Input: part model. Units: mm. Frame: model coordinates. A direction names the side the tool comes from. Round coordinates to 2 decimals unless told otherwise and drop trailing zeros. Order: outer loops, then holes, each group sorted by start corner. A loop starts at its lowest first (then second) coordinate and runs counter-clockwise, first axis right, second up. Notation, with made-up numbers: (57, 38) -> (91, 38) arc R25 cw to (91, 52) -> close; hole circle Ø2 at (11.25, 78). An arc over 180 degrees is marked (long way). Use a Markdown table: item, result.
from build123d import *

# Parameters (mm, degrees)
SKETCH_W                = 90
SKETCH_H                = 35
PAD_DEPTH               = 3
SKETCH001_R             = 10.5
HOLE_DEPTH              = 25
HOLE_TEARDROPS_DEPTH    = 25
SKETCH002_R             = 4
PAD001_DEPTH            = 5.6
POCKET_DEPTH            = 5.6
SKETCH004_R             = 1.45
HOLE001_DEPTH           = 25
HOLE001_TEARDROPS_DEPTH = 25
FILLET_R                = 2
CHAMFER_SIZE            = 0.4
FILLET001_R             = 1
PAD002_DEPTH            = 7
SKETCH005_R             = 14.71653
PAD003_DEPTH            = 10
SKETCH006_R             = 4.05
PAD004_DEPTH            = 5.6
POCKET001_DEPTH         = 5.6
SKETCH008_R             = 1.45
HOLE002_DEPTH           = 25
HOLE002_TEARDROPS_DEPTH = 25
FILLET002_R             = 2
CHAMFER001_SIZE         = 0.4
POCKET002_DEPTH         = 7
CHAMFER002_SIZE         = 0.4
CHAMFER003_SIZE         = 0.6


with BuildPart() as part:
    # Sketch → Pad (new body)
    with BuildSketch(Plane.XY):
        Rectangle(SKETCH_W, SKETCH_H)
    extrude(amount=PAD_DEPTH)

    # Sketch001 (on Face6 of Pad) → Hole (cut)
    with BuildSketch(Plane.XY.offset(3)):
        with Locations((-12, 0)):
            Circle(SKETCH001_R)
    extrude(amount=-HOLE_DEPTH, mode=Mode.SUBTRACT)

    # Sketch001_Teardrops (on Sketch) → Hole_Teardrops (cut)
    with BuildSketch(Plane.XY.offset(3)):
        with BuildLine():
            ThreePointArc((-17.25, 9.093267), (-12, -10.5), (-6.75, 9.093267))
            Line((-6.75, 9.093267), (-12, 12.124356))
            Line((-17.25, 9.093267), (-12, 12.124356))
        make_face()
    extrude(amount=-HOLE_TEARDROPS_DEPTH, mode=Mode.SUBTRACT)

    # Sketch002 (on Face5 of Hole_Teardrops) → Pad001 (join)
    with BuildSketch(Plane.XY.offset(3)):
        with Locations((35, 0)):
            Circle(SKETCH002_R)
        with Locations((12, 0)):
            Circle(SKETCH002_R)
        with Locations((-35, 0)):
            Circle(SKETCH002_R)
    extrude(amount=PAD001_DEPTH)

    # Sketch003 (on Face13 of Pad001) → Pocket (cut)
    with BuildSketch(Plane.XY.offset(8.6)):
        Polygon((-35, 3), (-38.464102, 5), (-31.535898, 5), align=None)
        Polygon((12, 3), (8.535898, 5), (15.464102, 5), align=None)
        Polygon((38.464102, 5), (35, 3), (31.535898, 5), align=None)
    extrude(amount=-POCKET_DEPTH, mode=Mode.SUBTRACT)

    # Sketch004 (on Face17 of Pocket) → Hole001 (cut)
    with BuildSketch(Plane.XY.offset(8.6)):
        with Locations((-35, 0)):
            Circle(SKETCH004_R)
        with Locations((12, 0)):
            Circle(SKETCH004_R)
        with Locations((35, 0)):
            Circle(SKETCH004_R)
    extrude(amount=-HOLE001_DEPTH, mode=Mode.SUBTRACT)

    # Sketch004_Teardrops (on Sketch) → Hole001_Teardrops (cut)
    with BuildSketch(Plane.XY.offset(8.6)):
        with BuildLine():
            ThreePointArc((-35.725, 1.255737), (-35, -1.45), (-34.275, 1.255737))
            Line((-34.275, 1.255737), (-35, 1.674316))
            Line((-35.725, 1.255737), (-35, 1.674316))
        make_face()
        with BuildLine():
            ThreePointArc((11.275, 1.255737), (12, -1.45), (12.725, 1.255737))
            Line((12.725, 1.255737), (12, 1.674316))
            Line((11.275, 1.255737), (12, 1.674316))
        make_face()
        with BuildLine():
            ThreePointArc((34.275, 1.255737), (35, -1.45), (35.725, 1.255737))
            Line((35.725, 1.255737), (35, 1.674316))
            Line((34.275, 1.255737), (35, 1.674316))
        make_face()
    extrude(amount=-HOLE001_TEARDROPS_DEPTH, mode=Mode.SUBTRACT)

    # Fillet
    fillet_edges = [part.edges().sort_by_distance(p)[0] for p in [
        (36.334875, 3.770691, 5.8),
        (33.665125, 3.770691, 5.8),
        (13.334875, 3.770691, 5.8),
        (10.665125, 3.770691, 5.8),
        (-33.665125, 3.770691, 5.8),
        (-36.334875, 3.770691, 5.8),
    ]]
    fillet(fillet_edges, radius=FILLET_R)

    # Chamfer
    chamfer_edges = [part.edges().sort_by_distance(p)[0] for p in [
        (33.392214, -3.662653, 8.6),
        (10.392214, -3.662653, 8.6),
        (-36.607786, -3.662653, 8.6),
        (-35.725, -1.255737, 8.6),
        (11.275, -1.255737, 8.6),
        (34.275, -1.255737, 8.6),
    ]]
    chamfer(chamfer_edges, length=CHAMFER_SIZE)

    # Fillet001
    fillet001_edges = [part.edges().sort_by_distance(p)[0] for p in [
        (45, 17.5, 1.5),
        (-45, 17.5, 1.5),
        (-45, -17.5, 1.5),
        (45, -17.5, 1.5),
    ]]
    fillet(fillet001_edges, radius=FILLET001_R)

    # Fillet001 Face28 → Pad002 (add)
    with BuildSketch(Plane(origin=(1.493435, -0.023344, 0), x_dir=(0, -1, 0), z_dir=(0, 0, -1))):
        with BuildLine():
            Line((16.476656, 46.493435), (-16.523344, 46.493435))
            ThreePointArc((-16.523344, 46.493435), (-17.230451, 46.200542), (-17.523344, 45.493435))
            Line((-17.523344, 45.493435), (-17.523344, -42.506565))
            ThreePointArc((-17.523344, -42.506565), (-17.230451, -43.213672), (-16.523344, -43.506565))
            Line((-16.523344, -43.506565), (16.476656, -43.506565))
            ThreePointArc((16.476656, -43.506565), (17.183762, -43.213672), (17.476656, -42.506565))
            Line((17.476656, -42.506565), (17.476656, 45.493435))
            ThreePointArc((17.476656, 45.493435), (17.183762, 46.200542), (16.476656, 46.493435))
        make_face()
        with BuildLine():
            ThreePointArc((-0.023344, 35.043435), (-0.748344, 35.237698), (-1.279081, 35.768435))
            Line((-1.279081, 35.768435), (-1.69766, 36.493435))
            Line((-1.69766, 36.493435), (-1.279081, 37.218435))
            ThreePointArc((-1.279081, 37.218435), (1.232392, 37.218435), (-0.023344, 35.043435))
        make_face(mode=Mode.SUBTRACT)
        with BuildLine():
            ThreePointArc((-0.023344, -11.956565), (-0.748344, -11.762302), (-1.279081, -11.231565))
            Line((-1.279081, -11.231565), (-1.69766, -10.506565))
            Line((-1.69766, -10.506565), (-1.279081, -9.781565))
            ThreePointArc((-1.279081, -9.781565), (1.232392, -9.781565), (-0.023344, -11.956565))
        make_face(mode=Mode.SUBTRACT)
        with BuildLine():
            ThreePointArc((-0.023344, -34.956565), (-0.748344, -34.762302), (-1.279081, -34.231565))
            Line((-1.279081, -34.231565), (-1.69766, -33.506565))
            Line((-1.69766, -33.506565), (-1.279081, -32.781565))
            ThreePointArc((-1.279081, -32.781565), (1.232392, -32.781565), (-0.023344, -34.956565))
        make_face(mode=Mode.SUBTRACT)
        with BuildLine():
            ThreePointArc((-0.023344, 2.993435), (-5.273344, 4.400168), (-9.116611, 8.243435))
            Line((-9.116611, 8.243435), (-12.1477, 13.493435))
            Line((-12.1477, 13.493435), (-9.116611, 18.743435))
            ThreePointArc((-9.116611, 18.743435), (9.069922, 18.743435), (-0.023344, 2.993435))
        make_face(mode=Mode.SUBTRACT)
    extrude(amount=PAD002_DEPTH)

    # Sketch005 (on Face3 of Pad002) → Pad003 (join)
    with BuildSketch(Plane.XY.offset(3)):
        with Locations((-11.639154, 0)):
            Circle(SKETCH005_R)
    extrude(amount=-PAD003_DEPTH)

    # Sketch006 (on Face67 of Pad003) → Pad004 (join)
    with BuildSketch(Plane.XY.offset(3)):
        with Locations((-12, 0)):
            Circle(SKETCH006_R)
    extrude(amount=PAD004_DEPTH)

    # Sketch007 (on Face66 of Pad004) → Pocket001 (cut)
    with BuildSketch(Plane.XY.offset(8.6)):
        Polygon((-12, 3), (-15.464102, 5), (-8.535898, 5), align=None)
    extrude(amount=-POCKET001_DEPTH, mode=Mode.SUBTRACT)

    # Sketch008 (on Face69 of Pocket001) → Hole002 (cut)
    with BuildSketch(Plane.XY.offset(8.6)):
        with Locations((-12, 0)):
            Circle(SKETCH008_R)
    extrude(amount=-HOLE002_DEPTH, mode=Mode.SUBTRACT)

    # Sketch008_Teardrops (on Sketch) → Hole002_Teardrops (cut)
    with BuildSketch(Plane.XY.offset(8.6)):
        with BuildLine():
            ThreePointArc((-12.725, 1.255737), (-12, -1.45), (-11.275, 1.255737))
            Line((-11.275, 1.255737), (-12, 1.674316))
            Line((-12.725, 1.255737), (-12, 1.674316))
        make_face()
    extrude(amount=-HOLE002_TEARDROPS_DEPTH, mode=Mode.SUBTRACT)

    # Fillet002
    fillet002_edges = [part.edges().sort_by_distance(p)[0] for p in [
        (-10.608429, 3.803424, 5.8),
        (-13.391571, 3.803424, 5.8),
    ]]
    fillet(fillet002_edges, radius=FILLET002_R)

    # Chamfer001
    chamfer001_edges = [part.edges().sort_by_distance(p)[0] for p in [
        (-12.725, -1.255737, 8.6),
        (-13.613716, -3.714623, 8.6),
    ]]
    chamfer(chamfer001_edges, length=CHAMFER001_SIZE)

    # Chamfer001 Face41 → Pocket002 (cut)
    with BuildSketch(Plane(origin=(0, -0.000217, -7), x_dir=(0, -1, 0), z_dir=(0, 0, -1))):
        with BuildLine():
            Line((16.499783, 45), (-16.500217, 45))
            ThreePointArc((-16.500217, 45), (-17.207324, 44.707107), (-17.500217, 44))
            Line((-17.500217, 44), (-17.500217, -44))
            ThreePointArc((-17.500217, -44), (-17.207324, -44.707107), (-16.500217, -45))
            Line((-16.500217, -45), (16.499783, -45))
            ThreePointArc((16.499783, -45), (17.20689, -44.707107), (17.499783, -44))
            Line((17.499783, -44), (17.499783, 44))
            ThreePointArc((17.499783, 44), (17.20689, 44.707107), (16.499783, 45))
        make_face()
        with BuildLine():
            ThreePointArc((-0.000217, -36.45), (-0.725217, -36.255737), (-1.255954, -35.725))
            Line((-1.255954, -35.725), (-1.674533, -35))
            Line((-1.674533, -35), (-1.255954, -34.275))
            ThreePointArc((-1.255954, -34.275), (1.25552, -34.275), (-0.000217, -36.45))
        make_face(mode=Mode.SUBTRACT)
        with BuildLine():
            ThreePointArc((-0.000217, -13.45), (-0.725217, -13.255737), (-1.255954, -12.725))
            Line((-1.255954, -12.725), (-1.674533, -12))
            Line((-1.674533, -12), (-1.255954, -11.275))
            ThreePointArc((-1.255954, -11.275), (1.25552, -11.275), (-0.000217, -13.45))
        make_face(mode=Mode.SUBTRACT)
        with BuildLine():
            ThreePointArc((-0.000217, 33.55), (-0.725217, 33.744263), (-1.255954, 34.275))
            Line((-1.255954, 34.275), (-1.674533, 35))
            Line((-1.674533, 35), (-1.255954, 35.725))
            ThreePointArc((-1.255954, 35.725), (1.25552, 35.725), (-0.000217, 33.55))
        make_face(mode=Mode.SUBTRACT)
        with BuildLine():
            ThreePointArc((-1.255954, 12.725), (1.25552, 12.725), (-0.000217, 10.55))
            ThreePointArc((-0.000217, 10.55), (-0.725217, 10.744263), (-1.255954, 11.275))
            Line((-1.255954, 11.275), (-1.674533, 12))
            Line((-1.674533, 12), (-1.255954, 12.725))
        make_face(mode=Mode.SUBTRACT)
    extrude(amount=-POCKET002_DEPTH, mode=Mode.SUBTRACT)

    # Chamfer002
    chamfer002_edges = [part.edges().sort_by_distance(p)[0] for p in [
        (0, -17.5, 3),
        (0, -17.5, 0),
    ]]
    chamfer(chamfer002_edges, length=CHAMFER002_SIZE)

    # Chamfer003
    chamfer003_edges = [part.edges().sort_by_distance(p)[0] for p in [
        (34.275, -1.255737, 0),
        (11.275, -1.255737, 0),
        (-12.725, -1.255737, 0),
        (-35.725, -1.255737, 0),
    ]]
    chamfer(chamfer003_edges, length=CHAMFER003_SIZE)


solid = part.part
1) Cut plane A-A on z = 5.5. Count the separate pieces of the cut face and the enclosed holes in it, and give its area (3 significant figures).
Results found:
| item | result |
|---|---|
| separate pieces | 4 |
| enclosed holes | 4 |
| area | 168 mm² |
2) Pull-direction query (Y, two-part tool) for faces 1 (the cylindrical face through (33.44, 3.46, 5.56)), 2 (the cylindrical face through (34.95, -1.45, 4.45)), 3 (the flat face through (45, 0, 2)), 4 (the cylindrical face through (-12.136, -4.048, 5.564)); classes: +Y half, -Y half, draft (parallel to the pull), parting line (faces both ways), or undercut.
Results found:
| item | result |
|---|---|
| face 1 | +Y half |
| face 2 | undercut |
| face 3 | draft |
| face 4 | parting line |
3) Cut plane C-C on x = -30. Return loops of the section in (y, z), and give its area (3 significant figures).
Results found:
| item | result |
|---|---|
| outline | (-17.5, 0.4) -> (-17.1, 0) -> (17.1, 0) -> (17.5, 0.4) -> (17.5, 2.6) -> (17.1, 3) -> (-17.1, 3) -> (-17.5, 2.6) -> close |
| area | 105 mm² |
4) Set-up query: faces 5 (the cylindrical face through (36.56, 3.46, 5.56)), 6 (the flat face through (-1, 0, 0)). Return all of +Z, -Z, +X, -X, +Y, -Y with unobstructed straight access to the full face (end or side cutting, diameter ignored); none if empty.
Results found:
| item | result |
|---|---|
| face 5 | +Z, +Y |
| face 6 | -Z, +X, -X, +Y, -Y |
5) Cut plane B-B on y = -14.5. Return loops of the section in (x, z).
Results found:
| item | result |
|---|---|
| outline | (-45, 0.4) -> (-44.6, 0) -> (44.6, 0) -> (45, 0.4) -> (45, 2.6) -> (44.6, 3) -> (-44.6, 3) -> (-45, 2.6) -> close |
6) Pin query (flat end, axial travel): pin 1 Ø1.5 at (x, z) = (16, 7.5) entering from -Y; pin 2 Ø3.5 at (x, y) = (35, 0) entering from +Z; pin 3 Ø3.5 at (x, y) = (-12, 0) entering from -Z. Return the tip coordinate at first contact, or that it passes through.
Results found:
| item | result |
|---|---|
| pin 1 | stops at y = -2.33 |
| pin 2 | stops at z = 8.5 |
| pin 3 | stops at z = 0.3 |
7) Line query: L1, parallel to Y at x = 12, z = 2.5; L2, parallel to Y at x = -12, z = 6.5; L3, parallel to Z at x = 30.5, y = 13. Output: solid intervals per line, ascending. Write a range as [from, to].
Results found:
| item | result |
|---|---|
| L1 | y = [-17.5, -1.45], [1.67, 17.5] |
| L2 | y = [-4.05, -1.45], [1.67, 3] |
| L3 | z = [0, 3] |
